Verification items for the finished model (mm, model axes). Give positions to 0.01 mm unless a question says otherwise; leave off trailing zeros. Write each loop counter-clockwise with the first axis right and the second up, starting at its lowest first coordinate (ties: lowest second). Pieces come first, ordered by that corner, then holes. Notation, with made-up numbers: (36.25, 58) - (84.25, 58) arc R29 ccw to (84.25, 92) - close; hole circle Ø2 at (3, -16). An arc over 180 degrees is marked (long way). Answer as a JSON object with one key per item and string values. Group by question number.
Item 1: Sectioned sample at B-B, the plane x = 0. Record the boundary of the cut face in (y, z).
Item 2: Go/stop test with flat-tipped pins: pin 1 (4 mm diameter, centred on y = -24.5, z = 3.5, fed in from -X); pin 2 (5 mm diameter, centred on x = 22, y = 36, fed in from -Z); pin 3 (4 mm diameter, centred on x = 17.5, z = 4.5, fed in from +Y); pin 4 (8.5 mm diameter, centred on x = 0, y = -41.68, fed in from -Z). Record where each tip stops, or that it passes through.
Item 3: Scan lines: line 1 along Y through (x, z) = (0.5, 9.5); line 2 along Y through (x, z) = (6, 11); line 3 along X through (y, z) = (46.5, 6.25). Record each from-to range of solid material in increasing order. Write a range as [from, to].
Item 4: Draft check along X on faces 1 (the face through (-1, -12, 12.7)), 2 (the face through (-0.621, 47.848, 6.261)), 3 (the face through (-12.39, -55.795, 6.261)). Enter one of: +X half, -X half, draft (parallel to the pull), parting line (faces both ways), or undercut.
Item 5: Sectioned sample at A-A, the plane y = 0. Record the boundary of the cut face in (x, z).
Item 6: Sectioned sample at D-D, the plane x = 49. Record the boundary of the cut face in (y, z), and give its area (3 significant figures).
Item 7: Sectioned sample at C-C, the plane z = 7.5. Record the boundary of the cut face in (x, y), and give its area (3 significant figures).
```python
from build123d import *

# Parameters (mm, degrees)
F0_R     = 57.153655
F0_R_2   = 4.759266
F0_R_3   = 4.767274
F0_R_4   = 9.529019
F0_R_5   = 4.758407
F0_R_6   = 4.76816
F1_DEPTH = 12.7


with BuildPart() as f1:
    # F0 (on Top) → F1 (new body)
    with BuildSketch(Plane.XY):
        Circle(F0_R)
        with Locations((0, -41.678783)):
            Circle(F0_R_2, mode=Mode.SUBTRACT)
        with Locations((-41.378908, 0)):
            Circle(F0_R_3, mode=Mode.SUBTRACT)
        Circle(F0_R_4, mode=Mode.SUBTRACT)
        with Locations((41.055638, 0)):
            Circle(F0_R_5, mode=Mode.SUBTRACT)
        with Locations((0, 43.120254)):
            Circle(F0_R_6, mode=Mode.SUBTRACT)
    extrude(amount=F1_DEPTH)


solid = f1.part
```
Geometry check:
{
 "1": {"outline": "(-57.15, 0) - (-46.44, 0) - (-46.44, 12.7) - (-57.15, 12.7) - close; (-36.92, 0) - (-9.53, 0) - (-9.53, 12.7) - (-36.92, 12.7) - close; (9.53, 0) - (38.35, 0) - (38.35, 12.7) - (9.53, 12.7) - close; (47.89, 0) - (57.15, 0) - (57.15, 12.7) - (47.89, 12.7) - close"},
 "2": {"pin 1": "x = -52.54", "pin 2": "z = 0", "pin 3": "y = 55.01", "pin 4": "through"},
 "3": {"line 1": "[-57.15, -46.41], [-36.95, -9.52], [9.52, 38.38], [47.86, 57.15]", "line 2": "[-56.84, -7.4], [7.4, 56.84]", "line 3": "[-33.23, -3.36], [3.36, 33.23]"},
 "4": {"face 1": "draft", "face 2": "undercut", "face 3": "parting line"},
 "5": {"outline": "(-57.15, 0) - (-46.15, 0) - (-46.15, 12.7) - (-57.15, 12.7) - close; (-36.61, 0) - (-9.53, 0) - (-9.53, 12.7) - (-36.61, 12.7) - close; (9.53, 0) - (36.3, 0) - (36.3, 12.7) - (9.53, 12.7) - close; (45.81, 0) - (57.15, 0) - (57.15, 12.7) - (45.81, 12.7) - close"},
 "6": {"outline": "(-29.42, 0) - (29.42, 0) - (29.42, 12.7) - (-29.42, 12.7) - close", "area": "747 mm^2"},
 "7": {"outline": "circle Ø114.31 at (0, 0); hole circle Ø9.53 at (-41.38, 0); hole circle Ø19.06 at (0, 0); hole circle Ø9.54 at (0, 43.12); hole circle Ø9.52 at (0, -41.68); hole circle Ø9.52 at (41.06, 0)", "area": "9,690 mm^2"}
}
